```python
from build123d import *

# Parameters (mm, degrees)
SKETCH1_W           = 105
SKETCH1_H           = 154
BOSS_EXTRUDE1_DEPTH = 5
SKETCH3_R           = 1.5
CUT_EXTRUDE1_DEPTH  = 10
SKETCH4_R           = 1.5
CUT_EXTRUDE2_DEPTH  = 6
SKETCH6_R           = 1.5
CUT_EXTRUDE4_DEPTH  = 6


with BuildPart() as part:
    # Sketch1 → Boss-Extrude1 (new body)
    with BuildSketch(Plane.XY):
        with Locations((12.5, -42)):
            Rectangle(SKETCH1_W, SKETCH1_H)
    extrude(amount=BOSS_EXTRUDE1_DEPTH)

    # Sketch3 → Cut-Extrude1 (cut)
    with BuildSketch(Plane(origin=(0, 0, 0), x_dir=(-1, 0, 0), z_dir=(0, 0, -1))):
        with Locations((32, -43)):
            Circle(SKETCH3_R)
        with Locations((32, -85)):
            Circle(SKETCH3_R)
        with Locations((3, -111)):
            Circle(SKETCH3_R)
        with Locations((3, -43)):
            Circle(SKETCH3_R)
        with Locations((32, -111)):
            Circle(SKETCH3_R)
        with Locations((3, -85)):
            Circle(SKETCH3_R)
        with Locations((3, -69)):
            Circle(SKETCH3_R)
        with Locations((32, -69)):
            Circle(SKETCH3_R)
    extrude(amount=-CUT_EXTRUDE1_DEPTH, mode=Mode.SUBTRACT)

    # Sketch4 → Cut-Extrude2 (cut, through all)
    with BuildSketch(Plane(origin=(0, 0, 0), x_dir=(-1, 0, 0), z_dir=(0, 0, -1))):
        with Locations((-25, 25)):
            Circle(SKETCH4_R)
        with Locations((25, 25)):
            Circle(SKETCH4_R)
        with Locations((25, -24.60667729)):
            Circle(SKETCH4_R)
        with Locations((-25, -24.60667729)):
            Circle(SKETCH4_R)
    extrude(amount=-CUT_EXTRUDE2_DEPTH, mode=Mode.SUBTRACT)

    # Sketch6 → Cut-Extrude4 (cut, through all)
    with BuildSketch(Plane(origin=(0, 0, 0), x_dir=(-1, 0, 0), z_dir=(0, 0, -1))):
        with Locations((-10, -47.56)):
            Circle(SKETCH6_R)
        with Locations((-55.018401793, -45.02)):
            Circle(SKETCH6_R)
        with Locations((-55.018401793, -99)):
            Circle(SKETCH6_R)
        with Locations((-10, -99)):
            Circle(SKETCH6_R)
    extrude(amount=-CUT_EXTRUDE4_DEPTH, mode=Mode.SUBTRACT)


solid = part.part
```
Could you check a few things on this model? Use its own coordinates, in mm. Round coordinates to 2 decimals unless told otherwise and drop trailing zeros. Order: outer loops, then holes, each group sorted by start corner. A loop starts at its lowest first (then second) coordinate and runs counter-clockwise, first axis right, second up. Notation, with made-up numbers: M -34.5,-30 L 12.5,-30 A15 ccw 12.5,-18 Z; hole C 45,53.25 d4. An arc over 180 degrees is marked long. One line per question, with ' | ' between items. Start each with the question number.
(1) Suppose I cut it at A-A on x = 10. List the corners of the cut face in (y, z) for me.
(2) Thinking about a two-plate mould opening in X: for faces 1 (the face through (-30.8, -43.9, 2.5)), 2 (the face through (65, -43, 2)), 3 (the face through (12, -41, 0)), 4 (the face through (-40, -43, 2)), which applies, +X half, -X half, draft (parallel to the pull), parting line (faces both ways), or undercut?
(3) Please list where these lines run through material, in increasing order: line 1 along Y through (x, z) = (-25, 3.1); line 2 along Y through (x, z) = (-3, 3.4); line 3 along Y through (x, z) = (-33, 4.35).
(4) Suppose I cut it at B-B on y = -85. List the corners of the cut face in (x, z) for me.
Geometry results:
1) outline: M -119,0 L -100.5,0 L -100.5,5 L -119,5 Z; M -97.5,0 L -49.06,0 L -49.06,5 L -97.5,5 Z; M -46.06,0 L 35,0 L 35,5 L -46.06,5 Z
2) face 1: undercut | face 2: +X half | face 3: draft | face 4: -X half
3) line 1: -119 to -26.11, -23.11 to 23.5, 26.5 to 35 | line 2: -119 to -112.5, -109.5 to -86.5, -83.5 to -70.5, -67.5 to -44.5, -41.5 to 35 | line 3: -119 to -112.12, -109.88 to -86.12, -83.88 to -70.12, -67.88 to -44.12, -41.88 to 35
4) outline: M -40,0 L -33.5,0 L -33.5,5 L -40,5 Z; M -30.5,0 L -4.5,0 L -4.5,5 L -30.5,5 Z; M -1.5,0 L 65,0 L 65,5 L -1.5,5 Z
